from build123d import *

# Parameters (mm, degrees)
SKETCH2_W               = 25.711141267
SKETCH2_H               = 16.935482271
CUT_REVOLVE1_ANGLE      = 270
SKETCH3_R               = 12.1123055
CUT_EXTRUDE1_DEPTH      = 12
CUT_EXTRUDE2_DEPTH      = 46.936892374
CUT_EXTRUDE2_DEPTH_BACK = 46.936892374


with BuildPart() as part:
    # Sketch1 → Revolve1 (revolve)
    with BuildSketch(Plane.XY):
        Polygon((-21.368212172, 15), (-21.368212172, 10), (21.368212172, 10), (21.368212172, 15), (37.560067367, 15), (37.560067367, 10), (45.936892374, 10), (45.936892374, 20), (-45.936892374, 20), (-45.936892374, 10), (-37.560067367, 10), (-37.560067367, 15), align=None)
    revolve(axis=Axis((-29.383970125, 0, 0), (1, 0, 0)))

    # Sketch2 → Cut-Revolve1 (revolve, symmetric, cut)
    with BuildSketch(Plane.XY) as cut_revolve1_sk:
        with Locations((-0.846360068, 17.320379596)):
            Rectangle(SKETCH2_W, SKETCH2_H)
    revolve(axis=Axis((-31.735702272, 0, 0), (1, 0, 0)), revolution_arc=CUT_REVOLVE1_ANGLE / 2, mode=Mode.SUBTRACT)
    revolve(cut_revolve1_sk.sketch, axis=Axis((-31.735702272, 0, 0), (-1, 0, 0)), revolution_arc=CUT_REVOLVE1_ANGLE / 2, mode=Mode.SUBTRACT)

    # Sketch3 → Cut-Extrude1 (cut)
    with BuildSketch(Plane.ZY.offset(45.936892374)):
        Circle(SKETCH3_R)
    cut_extrude1 = extrude(amount=-CUT_EXTRUDE1_DEPTH, mode=Mode.SUBTRACT)

    # Mirror1: Cut-Extrude1 across plane
    add(cut_extrude1.mirror(Plane(origin=(0, 0, 0), x_dir=(0, 0, 1), z_dir=(1, 0, 0))), mode=Mode.SUBTRACT)

    # Sketch4 → Cut-Extrude2 (cut, two sides)
    with BuildSketch(Plane(origin=(0, 0, 0), x_dir=(0, 0, -1), z_dir=(1, 0, 0))) as cut_extrude2_sk:
        Polygon((-23.278590176, -18.936948358), (32.516125961, -18.936948358), (-2.217008588, -46.464804995), align=None)
    extrude(amount=CUT_EXTRUDE2_DEPTH, mode=Mode.SUBTRACT)
    extrude(cut_extrude2_sk.sketch, amount=-CUT_EXTRUDE2_DEPTH_BACK, mode=Mode.SUBTRACT)


solid = part.part
Verification items for the finished model (mm, model axes). A direction names the side the tool comes from. Give positions to 0.01 mm unless a question says otherwise; leave off trailing zeros. Order: outer loops, then holes, each group sorted by start corner. A loop starts at its lowest first (then second) coordinate and runs counter-clockwise, first axis right, second up. Notation, with made-up numbers: (82.25, 13) -> (89.25, 13) arc R31 cw to (89.25, 48) -> close; hole circle Ø3 at (26, 53.5). An arc over 180 degrees is marked (long way). Answer as CSV lines item,"result".
Q1. Release check for a two-part mould opening along Y. For faces 5 (the flat face through (-45.937, 9, -9)), 6 (the cylindrical face through (0, -10, 0)), 7 (the cylindrical face through (-41.81, -7.37, -9.61)), 8 (the flat face through (-1, -11, 11)) record: +Y half, -Y half, draft (parallel to the pull), parting line (faces both ways), or undercut.
Solutions:
face 5,"draft"
face 6,"undercut"
face 7,"undercut"
face 8,"+Y half"
Q2. Sectioned sample at C-C on z = 0. Record the cut outline in (x, y).
Solutions:
outline,"(-45.94, -18.94) -> (45.94, -18.94) -> (45.94, -12.11) -> (37.56, -12.11) -> (37.56, -15) -> (21.37, -15) -> (21.37, -10) -> (-21.37, -10) -> (-21.37, -15) -> (-37.56, -15) -> (-37.56, -12.11) -> (-45.94, -12.11) -> close; (-45.94, 12.11) -> (-37.56, 12.11) -> (-37.56, 15) -> (-21.37, 15) -> (-21.37, 10) -> (-13.7, 10) -> (-13.7, 20) -> (-45.94, 20) -> close; (12.01, 10) -> (21.37, 10) -> (21.37, 15) -> (37.56, 15) -> (37.56, 12.11) -> (45.94, 12.11) -> (45.94, 20) -> (12.01, 20) -> close"
Q3. Sectioned sample at B-B on y = 0. Count the separate pieces of the cut face and the enclosed holes in it, plus the area to 3 significant figures.
Solutions:
separate pieces,"4"
enclosed holes,"0"
area,"929 mm²"
Q4. Depth check by flat-ended pin: pin 1 (4 mm diameter, centred on x = 12, z = 10.5, fed in from -Y); pin 2 (16 mm diameter, centred on y = 0, z = 0, fed in from +X); pin 3 (17 mm diameter, centred on y = -3.5, z = 4, fed in from +X); pin 4 (1 mm diameter, centred on x = -7, y = -9.5, fed in from -Z). Enter the tip coordinate at first touch or a pass-through.
Solutions:
pin 1,"stops at y = -18.1"
pin 2,"passes through"
pin 3,"stops at x = 45.94"
pin 4,"stops at z = -10"
Q5. Sectioned sample at A-A on z = 16. Record the cut outline in (x, y), plus the area to 3 significant figures.
Solutions:
outline,"(-45.94, -12) -> (-13.7, -12) -> (-13.7, 12) -> (-45.94, 12) -> close; (12.01, -12) -> (45.94, -12) -> (45.94, 12) -> (12.01, 12) -> close"
area,"1,590 mm²"
Q6. Scan lines: probe 1 along X at (y, z) = (-9, 11); probe 2 along X at (y, z) = (9.5, 14); probe 3 along X at (y, z) = (-13.5, -3.5). Record each from-to range of solid material in increasing order.
Solutions:
probe 1,"x = -45.94 to -37.56, -21.37 to -13.7, 12.01 to 21.37, 37.56 to 45.94"
probe 2,"x = -45.94 to -13.7, 12.01 to 45.94"
probe 3,"x = -45.94 to -37.56, -21.37 to 21.37, 37.56 to 45.94"
Q7. Access from +Z, -Z, +X, -X, +Y, -Y to the whole of each face (thin tool, end or side, straight path). Record for faces 1 (the cylindrical face through (41.81, -7.37, -9.61)), 2 (the flat face through (-1, -11, -11)), 3 (the cylindrical face through (-29.351, -14.985, 0.66)), 4 (the cylindrical face through (-0.643, -15.557, 12.569)).
Solutions:
face 1,"+X"
face 2,"-Z, +Y"
face 3,"none"
face 4,"+X, -X"
Q8. Sectioned sample at D-D on y = 11. Record the cut outline in (x, z).
Solutions:
outline,"(-45.94, -16.7) -> (-13.7, -16.7) -> (-13.7, 16.7) -> (-45.94, 16.7) -> (-45.94, 5.07) -> (-37.56, 5.07) -> (-37.56, 10.2) -> (-21.37, 10.2) -> (-21.37, -10.2) -> (-37.56, -10.2) -> (-37.56, -5.07) -> (-45.94, -5.07) -> close; (12.01, -16.7) -> (45.94, -16.7) -> (45.94, -5.07) -> (37.56, -5.07) -> (37.56, -10.2) -> (21.37, -10.2) -> (21.37, 10.2) -> (37.56, 10.2) -> (37.56, 5.07) -> (45.94, 5.07) -> (45.94, 16.7) -> (12.01, 16.7) -> close"
